```python
from build123d import *

# Parameters (mm, degrees)
F0_W     = 50.8
F0_H     = 50.8
F1_DEPTH = 50.8
F2_W     = 25.4
F2_H     = 25.4
F3_DEPTH = 25.4
F4_W     = 25.4
F4_H     = 25.4
F5_DEPTH = 50.801


with BuildPart() as f1:
    # F0 (on Front) → F1 (new body)
    with BuildSketch(Plane.XZ):
        Rectangle(F0_W, F0_H)
    extrude(amount=F1_DEPTH)

    # F2 (on face) → F3 (join)
    with BuildSketch(Plane.XZ.offset(50.8)):
        Rectangle(F2_W, F2_H)
    extrude(amount=F3_DEPTH)

    # F4 (on face) → F5 (cut, through all)
    with BuildSketch(Plane.YZ.offset(25.4)):
        with Locations((-25.4, 0)):
            Rectangle(F4_W, F4_H)
    extrude(amount=-F5_DEPTH, mode=Mode.SUBTRACT)


solid = f1.part
```
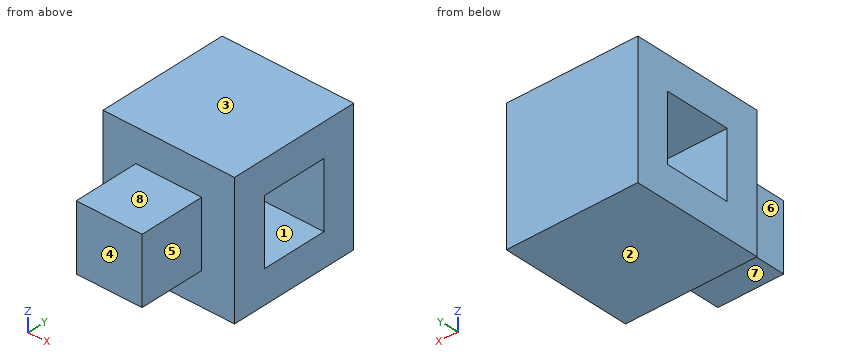
Input: part model. Units: mm. Frame: model coordinates. Face numbers are marked on the shaded views. A direction names the side the tool comes from. Give positions to 0.01 mm unless a question says otherwise; leave off trailing zeros. Loops run counter-clockwise (first coordinate to the right, second up) from the corner with the lowest first, then second, coordinate; pieces in that order, holes last. Notation, with made-up numbers: (47.5, 2.25) -> (51.5, 2.25) arc R19 ccw to (51.5, 30.25) -> close; hole circle Ø10 at (29, 17.25). An arc over 180 degrees is marked (long way). Use a Markdown table: item, result.
Q1. Section query C-C, the plane x = 9. Return the cut outline in (y, z), plus the area to 3 significant figures.
Entries:
| item | result |
|---|---|
| outline | (-76.2, -12.7) -> (-50.8, -12.7) -> (-50.8, -25.4) -> (0, -25.4) -> (0, 25.4) -> (-50.8, 25.4) -> (-50.8, 12.7) -> (-76.2, 12.7) -> close; hole (-38.1, -12.7) -> (-12.7, -12.7) -> (-12.7, 12.7) -> (-38.1, 12.7) -> close |
| area | 2,580 mm² |
Q2. Access query for the marked faces 5, 6, 7 and 8. Directions: +Z, -Z, +X, -X, +Y, -Y. A direction counts if a zero-diameter tool reaches every point of the face in a straight line with its end or side. Return the directions, or none.
Entries:
| item | result |
|---|---|
| face 5 | +Z, -Z, +X, -Y |
| face 6 | +Z, -Z, -X, -Y |
| face 7 | -Z, +X, -X, -Y |
| face 8 | +Z, +X, -X, -Y |
Q3. Pull-direction query (Z, two-part tool) for the marked faces 1, 2, 3 and 4; classes: pulls with the +Z half, pulls with the -Z half, needs draft (parallel to the pull), parting line crosses it, or undercut.
Entries:
| item | result |
|---|---|
| face 1 | undercut |
| face 2 | pulls with the -Z half |
| face 3 | pulls with the +Z half |
| face 4 | needs draft |
Q4. Ray query, probe 1 along Y at (x, z) = (-8, -3); probe 2 along Z at (x, y) = (19.5, -18.5); probe 3 along Y at (x, z) = (-18, -5.5). Return the intervals inside material, ascending. Write a range as from..to.
Entries:
| item | result |
|---|---|
| probe 1 | y = -76.2..-38.1, -12.7..0 |
| probe 2 | z = -25.4..-12.7, 12.7..25.4 |
| probe 3 | y = -50.8..-38.1, -12.7..0 |
Q5. Section query A-A, the plane z = -4. Return the cut outline in (x, y).
Entries:
| item | result |
|---|---|
| outline | (-25.4, -50.8) -> (-12.7, -50.8) -> (-12.7, -76.2) -> (12.7, -76.2) -> (12.7, -50.8) -> (25.4, -50.8) -> (25.4, -38.1) -> (-25.4, -38.1) -> close; (-25.4, -12.7) -> (25.4, -12.7) -> (25.4, 0) -> (-25.4, 0) -> close |
Q6. Section query B-B, the plane y = -16. Return the cut outline in (x, z), plus the area to 3 significant figures.
Entries:
| item | result |
|---|---|
| outline | (-25.4, -25.4) -> (25.4, -25.4) -> (25.4, -12.7) -> (-25.4, -12.7) -> close; (-25.4, 12.7) -> (25.4, 12.7) -> (25.4, 25.4) -> (-25.4, 25.4) -> close |
| area | 1,290 mm² |
Q7. Section query D-D, the plane x = 19.5. Return the cut outline in (y, z), plus the area to 3 significant figures.
Entries:
| item | result |
|---|---|
| outline | (-50.8, -25.4) -> (0, -25.4) -> (0, 25.4) -> (-50.8, 25.4) -> close; hole (-38.1, -12.7) -> (-12.7, -12.7) -> (-12.7, 12.7) -> (-38.1, 12.7) -> close |
| area | 1,940 mm² |
Q8. First-contact query: P1, Ø10, axis at x = 20, z = -18.5, coming from the -Y side; P2, Ø10, axis at x = -13.5, y = -60, coming from the +Z side; P3, Ø12, axis at x = -15, y = -68, coming from the -Z side; P4, Ø8, axis at y = -33, z = -4, coming from the -X side. Flat tips, straight axial feed; report the tip coordinate or a pass-through.
Entries:
| item | result |
|---|---|
| P1 | stops at y = -50.8 |
| P2 | stops at z = 12.7 |
| P3 | stops at z = -12.7 |
| P4 | passes through |
